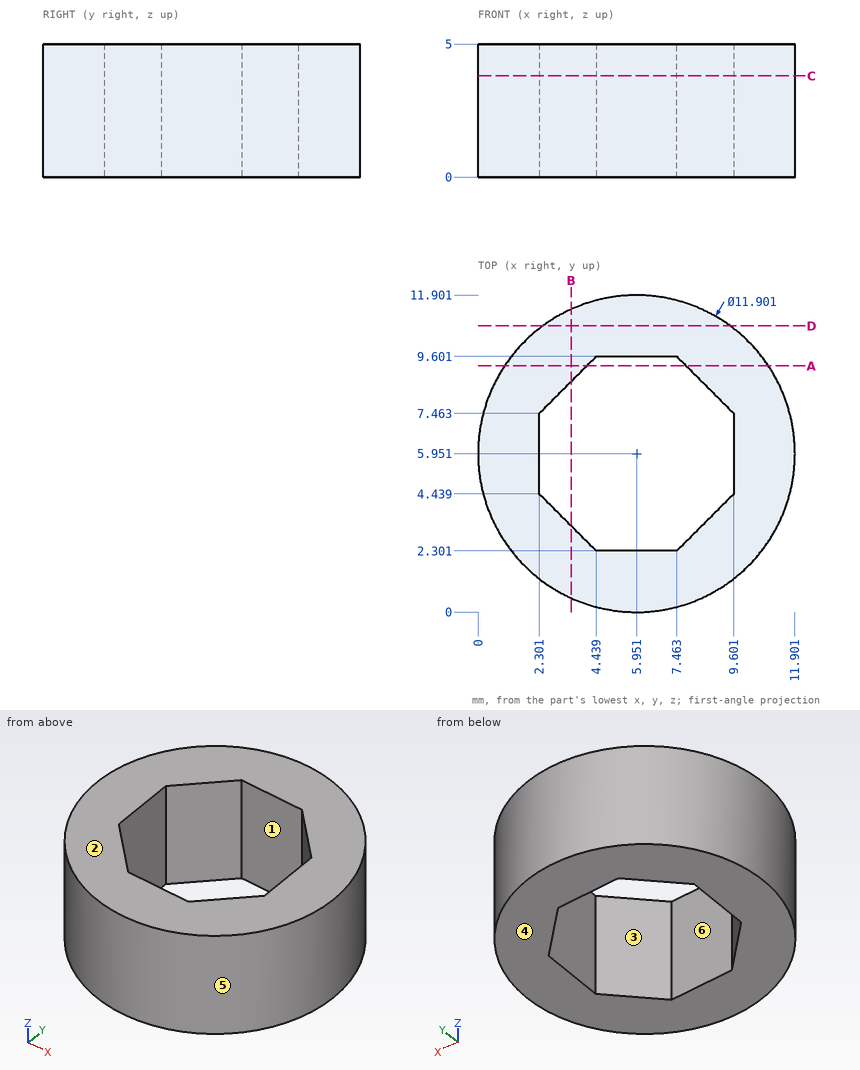
Drawing for the job (mm, zero at the part's lowest x, y, z). A direction names the side the tool comes from. Round coordinates to 2 decimals unless told otherwise and drop trailing zeros. Loops run counter-clockwise (first coordinate to the right, second up) from the corner with the lowest first, then second, coordinate; pieces in that order, holes last. Notation, with made-up numbers: (-39, -18.5) -> (-6, -18.5) arc R21 ccw to (-6, 3.5) -> close; hole circle Ø6 at (45, 35.25). An arc over 180 degrees is marked (long way). Answer in a Markdown table with one row per item.
Item 1: Saw through at B-B (x = 3.5). Write the cut outline in (y, z), and give its area (3 significant figures).
Answers below:
| item | result |
|---|---|
| outline | (0.53, 0) -> (3.24, 0) -> (3.24, 5) -> (0.53, 5) -> close; (8.66, 0) -> (11.37, 0) -> (11.37, 5) -> (8.66, 5) -> close |
| area | 27.1 mm² |
Item 2: Saw through at A-A (y = 9.25). Write the cut outline in (x, z), and give its area (3 significant figures).
Answers below:
| item | result |
|---|---|
| outline | (1, 0) -> (4.09, 0) -> (4.09, 5) -> (1, 5) -> close; (7.81, 0) -> (10.9, 0) -> (10.9, 5) -> (7.81, 5) -> close |
| area | 30.9 mm² |
Item 3: Mould opens along X. For the marked faces 3, 4, 5 and 6 say: +X half, -X half, draft (parallel to the pull), parting line (faces both ways), or undercut.
Answers below:
| item | result |
|---|---|
| face 3 | undercut |
| face 4 | draft |
| face 5 | parting line |
| face 6 | undercut |
Item 4: Pin check, flat tips, straight feed: pin 1 (2 mm diameter, centred on y = 3.5, z = 3.5, fed in from -X); pin 2 (1.5 mm diameter, centred on y = 4.5, z = 0.5, fed in from +X). Stop position of each tip, or through.
Answers below:
| item | result |
|---|---|
| pin 1 | stops at x = 0.18 |
| pin 2 | stops at x = 11.86 |
Item 5: Saw through at D-D (y = 10.75). Write the cut outline in (x, z).
Answers below:
| item | result |
|---|---|
| outline | (2.43, 0) -> (9.47, 0) -> (9.47, 5) -> (2.43, 5) -> close |
Item 6: Which spindle directions (+Z, -Z, +X, -X, +Y, -Y) get a long thin tool onto all of the face, cutting with end or side? Do the marked faces 1 and 2. Say none if no direction does.
Answers below:
| item | result |
|---|---|
| face 1 | +Z, -Z |
| face 2 | +Z, +X, -X, +Y, -Y |
Item 7: Drill centre lines: L1, parallel to X at y = 5.75, z = 0.3; L2, parallel to X at y = 2.5, z = 0.45 (1 decimal). Where is each one in solid material? Low to high. Write a range as [from, to].
Answers below:
| item | result |
|---|---|
| L1 | x = [0, 2.3], [9.6, 11.9] |
| L2 | x = [1.1, 4.2], [7.7, 10.8] |
Item 8: Saw through at C-C (z = 3.8). Write the cut outline in (x, y).
Answers below:
| item | result |
|---|---|
| outline | circle Ø11.9 at (5.95, 5.95); hole (2.3, 4.44) -> (4.44, 2.3) -> (7.46, 2.3) -> (9.6, 4.44) -> (9.6, 7.46) -> (7.46, 9.6) -> (4.44, 9.6) -> (2.3, 7.46) -> close |
